Here's how the part is built. I have some questions about the finished solid (model axes, mm). A direction names the side the tool comes from. Round coordinates to 2 decimals unless told otherwise and drop trailing zeros. Write each loop counter-clockwise with the first axis right and the second up, starting at its lowest first coordinate (ties: lowest second). Pieces come first, ordered by that corner, then holes. Notation, with made-up numbers: (-37.5, 4) - (-6.5, 4) arc R31 cw to (-6.5, 29) - close; hole circle Ø9 at (81.5, -11.75). An arc over 180 degrees is marked (long way). One line per item, written item: value. Start each with the question number.
Item 1: For faces 1 (the face through (-0.63, 7.85, 18.29)), 2 (the face through (7, 0, 15)), 3 (the face through (-3, 6, 15)), 4 (the face through (-6.336, -4.52, 15.143)), 5 (the face through (-3, -6, 15)), which set-ups out of +Z, -Z, +X, -X, +Y, -Y let a thin tool reach every point of the face, with its end or its side?
Item 2: Imagine slicing it at C-C, the plane x = -9. Please give me the cut outline in (y, z).
Item 3: For P1, Ø6, axis at y = 0, z = 18.5, coming from the +X side; P2, Ø2.5, axis at x = 0, y = 0, coming from the -Z side; P3, Ø0.6, axis at x = 7, y = 0, coming from the -Z side; P4, Ø1.2, axis at x = 6.5, z = 19, coming from the +Y side, each with a flat end and sliding along its axis, tell me the tip position at first contact or that it passes through.
Item 4: If I drill on line 1 (Y direction, x = 0, z = 15.5) (3 decimals); line 2 (Y direction, x = -6.5, z = 20.75); line 3 (Z direction, x = 10.25, y = 3.5), over which ranges is the centre line in solid material (lowest first)?
Item 5: Imagine slicing it at D-D, the plane y = 10. Please give me the cut outline in (x, z), then the cut area to 3 significant figures.
Item 6: Thinking about a two-plate mould opening in X: for faces 6 (the face through (3.11, 2.43, 17.53)), 7 (the face through (5.85, 0, 8)), 8 (the face through (2.15, 0.09, 3.94)), 9 (the face through (0, -3, 0)), which applies, released by +X, released by -X, zero draft, split by the parting line, or undercut?
Item 7: Imagine slicing it at A-A, the plane y = 0. Please give me the cut outline in (x, z), then the cut area to 3 significant figures.
Autodesk Inventor part; units mm, degrees
ref_plane "YZ Plane" through (0, 0, 0) normal (1, 0, 0) x (0, 1, 0)
ref_plane "XZ Plane" through (0, 0, 0) normal (0, 1, 0) x (-1, 0, 0)
ref_plane "XY Plane" through (0, 0, 0) normal (0, 0, 1) x (1, 0, 0)
sketch "草圖1" plane through (0, 0, 0) normal (0, 0, 1) x (1, 0, 0)
  line L0 (-5.85, 3.3775) -> (0, 6.755)
  line L1 (0, 6.755) -> (5.85, 3.3775)
  line L2 (5.85, 3.3775) -> (5.85, -3.3775)
  line L3 (5.85, -3.3775) -> (0, -6.755)
  line L4 (0, -6.755) -> (-5.85, -3.3775)
  line L5 (-5.85, -3.3775) -> (-5.85, 3.3775)
  point P0 (0, 0)
  point P1 (0, 0)
  dimension "d0" = 11.7
extrude "擠出1" add sketch "草圖1" along normal blind 24
sketch "草圖2" plane through (0, 0, 24) normal (0, 0, 1) x (1, 0, 0)
  circle A0 centre (0, 0) radius 14.25
  dimension "d3" = 28.5
extrude "擠出2" add sketch "草圖2" against normal blind 3
sketch "草圖3" plane through (0, 0, 21) normal (0, 0, -1) x (-1, 0, 0)
  line L0 (5.85, -3.3775) -> (0, -6.755)
  line L1 (5.85, 3.3775) -> (5.85, -3.3775)
  line L2 (0, 6.755) -> (5.85, 3.3775)
  line L3 (-5.85, 3.3775) -> (0, 6.755)
  line L4 (-5.85, -3.3775) -> (-5.85, 3.3775)
  line L5 (0, -6.755) -> (-5.85, -3.3775)
  line L6 (-5.85, 3.3775) -> (0, 6.755)
  line L7 (0, 6.755) -> (5.85, 3.3775)
  line L8 (0, 6.755) -> (5.85, 3.3775)
  line L9 (5.85, 3.3775) -> (7.1, 5.5426)
  line L10 (7.1, 5.5426) -> (1.25, 8.9201)
  line L11 (1.25, 8.9201) -> (0, 6.755)
  line L12 (-5.85, -3.3775) -> (-5.85, 3.3775)
  line L13 (-5.85, 3.3775) -> (-8.35, 3.3775)
  line L14 (-8.35, 3.3775) -> (-8.35, -3.3775)
  line L15 (-8.35, -3.3775) -> (-5.85, -3.3775)
  line L16 (5.85, -3.3775) -> (0, -6.755)
  line L17 (0, -6.755) -> (1.25, -8.9201)
  line L18 (1.25, -8.9201) -> (7.1, -5.5426)
  line L19 (7.1, -5.5426) -> (5.85, -3.3775)
  point P0 (0, 0)
  point P1 (0, -6.755)
  dimension "d6" = 2.5
  dimension "d9" = 360
extrude "擠出3" add sketch "草圖3" along normal blind 6 contours L19 L18 L17 L0 | L2 L11 L10 L9 | L15 L14 L13 L4
sketch "草圖4" plane through (0, 0, 0) normal (0, 0, -1) x (-1, 0, 0)
  circle A0 centre (0, 0) radius 2.1
  dimension "d13" = 4.2
extrude "擠出4" cut sketch "草圖4" against normal up to surface (24 mm away)
sketch "草圖5" plane through (0, 0, 0) normal (0, 0, -1) x (-1, 0, 0)
  circle A0 centre (0, 0) radius 2.1
  circle A1 centre (0, 0) radius 2.15
  dimension "d16" = 4.3
extrude "擠出5" cut sketch "草圖5" against normal blind 8 contours A0 | A1
sketch "草圖6" plane through (5.85, 3.3775, 15) normal (0.5, 0.866, 0) x (0.866, -0.5, 0)
  line L0 (10.8725, -6) -> (-17.6275, -6)
  circle A0 centre (-3.3775, -3) radius 1.5
  line L1 (-3.3775, 19.8) -> (-3.3775, -13.8)
  point P0 (-3.3775, 15)
  dimension "d19" = 3
  dimension "d22" = 3
extrude "擠出6" cut sketch "草圖6" against normal blind 6
sketch "草圖7" plane through (5.85, 3.3775, 15) normal (0.5, 0.866, 0) x (0.866, -0.5, 0)
  circle A0 centre (-3.3775, -3) radius 1.5
  circle A1 centre (-3.3775, -3) radius 1.55
  point P0 (-3.3775, 15)
  dimension "d23" = 3.1
extrude "擠出7" cut sketch "草圖7" against normal blind 6 contours A0 | A1
fillet "圓角2" radius 0.5 9 edges at (-4.175, 7.2313, 15) (-0.625, 7.8375, 15) (-6.475, 4.46, 15) (7.1, 3.3775, 15) (8.35, 0, 15) (7.1, -3.3775, 15) (-4.175, -7.2313, 15) (-0.625, -7.8375, 15) (-6.475, -4.46, 15)
properties part number "Coupling_0515"
Values follow:
1. face 1: -Z, +X, +Y
1. face 2: -Z, +X, +Y, -Y
1. face 3: -Z, -X, +Y
1. face 4: -Z, -X
1. face 5: -Z, -X, -Y
2. outline: (-11.05, 21) - (11.05, 21) - (11.05, 24) - (-11.05, 24) - close
3. P1: stops at x = 14.25
3. P2: passes through
3. P3: stops at z = 15
3. P4: stops at y = 3.38
4. line 1: y = -6.755 to -2.1, 2.1 to 6.755
4. line 2: y = -5.89 to -4.5, 4.5 to 5.89
4. line 3: z = 21 to 24
5. outline: (-10.15, 21) - (10.15, 21) - (10.15, 24) - (-10.15, 24) - close
5. area: 60.9 mm^2
6. face 6: undercut
6. face 7: released by +X
6. face 8: undercut
6. face 9: zero draft
7. outline: (-14.25, 21) - (-5.85, 21) - (-5.85, 0) - (-2.15, 0) - (-2.15, 8) - (-2.1, 8) - (-2.1, 24) - (-14.25, 24) - close; (2.1, 8) - (2.15, 8) - (2.15, 0) - (5.85, 0) - (5.85, 15) - (7.85, 15) arc R0.5 ccw to (8.35, 15.5) - (8.35, 21) - (14.25, 21) - (14.25, 24) - (2.1, 24) - close
7. area: 245 mm^2
